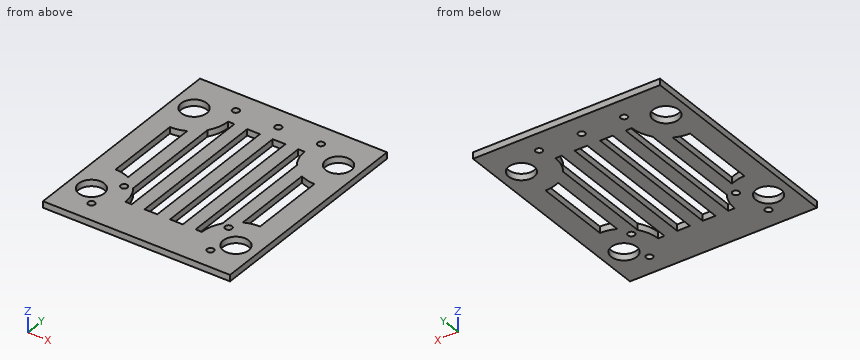
Autodesk Inventor part; units mm, degrees
ref_plane "YZ Plane" through (0, 0, 0) normal (1, 0, 0) x (0, 1, 0)
ref_plane "XZ Plane" through (0, 0, 0) normal (0, 1, 0) x (-1, 0, 0)
ref_plane "XY Plane" through (0, 0, 0) normal (0, 0, 1) x (1, 0, 0)
sketch "スケッチ1" plane through (0, 0, 0) normal (0, 0, 1) x (1, 0, 0)
  line L0 (-22, -24) -> (22, -24)
  line L1 (22, -24) -> (22, 24)
  line L2 (22, 24) -> (-22, 24)
  line L3 (-22, 24) -> (-22, -24)
  line L4 (-22, -24) -> (22, 24) construction
  line L5 (22, -24) -> (-22, 24) construction
  line L6 (-17, 15) -> (17, 15)
  line L7 (17, 15) -> (17, -19)
  line L8 (17, -19) -> (-17, -19)
  line L9 (-17, -19) -> (-17, 15)
  circle A0 centre (-17, 15) radius 3
  circle A1 centre (17, 15) radius 3
  circle A2 centre (17, -19) radius 3
  circle A3 centre (-17, -19) radius 3
  circle A4 centre (-17, 15) radius 8
  circle A5 centre (17, 15) radius 8
  circle A6 centre (17, -19) radius 8
  circle A7 centre (-17, -19) radius 8
  line L10 (-22, -24) -> (22, -24)
  line L11 (22, -24) -> (22, -28)
  line L12 (22, -28) -> (-22, -28)
  line L13 (-22, -28) -> (-22, -24)
  line L14 (-1.5, 15) -> (1.5, 15)
  line L15 (1.5, 15) -> (1.5, -19)
  line L16 (1.5, -19) -> (-1.5, -19)
  line L17 (-1.5, -19) -> (-1.5, 15)
  line L18 (7.5, 15) -> (7.5, -19)
  line L19 (4.5, -19) -> (4.5, 15)
  line L20 (13.5, 15) -> (13.5, -19)
  line L21 (10.5, -19) -> (10.5, 15)
  line L22 (-4.5, 15) -> (-4.5, -19)
  line L23 (-7.5, -19) -> (-7.5, 15)
  line L24 (1.5, 15) -> (1.5, -19)
  line L25 (-1.5, -19) -> (-1.5, 15)
  line L26 (7.5, 15) -> (7.5, -19)
  line L27 (4.5, -19) -> (4.5, 15)
  line L28 (-10.5, 15) -> (-10.5, -19)
  line L29 (-13.5, -19) -> (-13.5, 15)
  line L30 (-4.5, 15) -> (-4.5, -19)
  line L31 (-7.5, -19) -> (-7.5, 15)
  line L32 (1.5, 15) -> (1.5, -19)
  line L33 (-1.5, -19) -> (-1.5, 15)
  point P0 (0, 0)
  point P1 (-9, 15)
  point P2 (9, 15)
  point P3 (17, 7)
  point P4 (17, -11)
  point P5 (9, -19)
  point P6 (-9, -19)
  point P7 (-17, -11)
  point P8 (-17, 7)
  point P9 (22, -24)
  point P10 (0, 15)
  point P11 (-13.5, 7.8063)
  point P12 (-13.5, -11.8063)
  point P13 (-10.5, -14.3363)
  point P14 (-10.5, 10.3363)
  point P15 (10.5, 10.3363)
  point P16 (10.5, -14.3363)
  point P17 (13.5, -11.8063)
  point P18 (13.5, 7.8063)
  dimension "d0" = 48
  dimension "d1" = 44
  dimension "d2" = 34
  dimension "d3" = 5
  dimension "d4" = 5
  dimension "d5" = 6
  dimension "d6" = 16
  dimension "d11" = 4
  dimension "d12" = 3
  dimension "d15" = 6
  dimension "d18" = 6
extrude "プレート1" add sketch "スケッチ1" along normal blind 1.5 contours L3 A7 L9 A3 L8 L0 | L0 A7 L13 | A7 L8 A6 L0 | L0 A6 L11 L12 L13 A7 | L3 A4 L9 A7 | A6 L8 A2 L7 L1 L0 | L0 L11 A6 | L8 L28 A7 | L3 A4 L6 A0 L9 | A7 L29 L8 A3 L9 | A6 L21 L8 | L23 L6 L22 L8 | L8 L29 A7 L28 | A7 L29 A4 L28 | L3 L2 L1 A5 L6 A4 | L9 A0 L6 L29 A4 | A6 L7 A5 L1 | L21 A6 L20 L8 | L8 L19 L6 L18 | L21 A5 L20 A6 | L28 L6 A4 | A4 L29 L6 L28 | A5 L7 A1 L6 L1 | L7 A2 L8 L20 A6 | L21 L6 L20 A5 | A5 L6 L21 | L17 L6 L15 L8 | A5 L20 L6 A1 L7
sketch "スケッチ2" plane through (0, 0, 1.5) normal (0, 0, 1) x (1, 0, 0)
  line L0 (11.5, -21.5) -> (11.5, -14.8)
  line L1 (11.5, -21.5) -> (12, -21.5)
  line L2 (12, -21.5) -> (12, -24)
  line L3 (18, -24) -> (14, -24)
  line L4 (18, -14) -> (18, -24) construction
  line L5 (12.3, -14) -> (18, -14)
  circle A0 centre (12.3, -14.8) radius 0.8
  circle A1 centre (14, -23.2) radius 0.8
  line L6 (0, 0) -> (0, -10)
  circle A2 centre (-12.3, -14.8) radius 0.8
  circle A3 centre (-14, -23.2) radius 0.8
  arc A4 (11.5, -14.8) -> (12.3, -14) centre (12.3, -14.8) ccw
  line L7 (14, -24) -> (12, -24)
  circle A5 centre (14, -23.2) radius 0.8
  dimension "d21" = 1.6
  dimension "d22" = 1.6
  dimension "d25" = 2
extrude "切り取り1" cut sketch "スケッチ2" against normal blind 1.5
sketch "スケッチ3" plane through (0, 0, 1.5) normal (0, 0, 1) x (1, 0, 0)
  circle A0 centre (0, 19) radius 0.8
  circle A1 centre (-10, 19) radius 0.8
  circle A2 centre (10, 19) radius 0.8
  line L0 (-22, 24) -> (22, 24)
  point P0 (0, 0)
  point P1 (0, 24)
  dimension "d26" = 1.6
  dimension "d27" = 1.6
  dimension "d28" = 1.6
  dimension "d29" = 5
  dimension "d30" = 10
  dimension "d31" = 10
extrude "切り取り2" cut sketch "スケッチ3" against normal blind 1.5
equation "\"d4\" = d3"
equation "\"d23\" = Thickness"
equation "\"d32\" = Thickness"
equation "\"d10\" = Thickness"
equation "\"BendRadius\" = Thickness"
equation "\"BendReliefWidth\" = Thickness"
equation "\"BendReliefDepth\" = 0.5 * Thickness"
equation "\"CornerReliefSize\" = 4 * Thickness"
equation "\"MinimumRemnant\" = 2 * Thickness"
equation "\"TransitionRadius\" = BendRadius"
equation "\"JacobiRadiusSize\" = BendRadius"
equation "\"GapSize\" = Thickness"
properties part number "board_setter_base" material "アルミニウム 6061"
Geometry: final body of the model. Coordinates: model frame, mm. Coordinates: 2 decimals unless noted, no trailing zeros. Loops run counter-clockwise (first coordinate to the right, second up) from the corner with the lowest first, then second, coordinate; pieces in that order, holes last. Notation, with made-up numbers: (70.25, 60) - (88.25, 60) arc R25 cw to (88.25, 86) - close; hole circle Ø1 at (63, 3.5). An arc over 180 degrees is marked (long way). Put each result on its own line as item: value. Start each with the question number.
Q1. Line query: line 1 (X direction, y = 10, z = 0.2); line 2 (Y direction, x = -14.5, z = 0.45); line 3 (Y direction, x = 0, z = 0.55). Output: solid intervals per line, ascending.
Q2. Cut plane A-A, the plane x = -3.5. Return loops of the section in (y, z).
Q3. Cut plane D-D, the plane x = 18. Return loops of the section in (y, z), and give its area (3 significant figures).
Q4. Cut plane C-C, the plane y = -7. Return loops of the section in (x, z).
Q5. Pin query (flat end, axial travel): pin 1 Ø5.5 at (x, y) = (17, -19) entering from -Z. Return the tip coordinate at first contact, or that it passes through.
Q6. Cut plane B-B, the plane y = -23.2. Return loops of the section in (x, z).
Filled sheet:
1. line 1: -22 to -10.5, -7.5 to -4.5, -1.5 to 1.5, 4.5 to 7.5, 10.5 to 22
1. line 2: -28 to -23.82, -22.58 to -20.66, -17.34 to -11.4, 7.4 to 13.34, 16.66 to 24
1. line 3: -28 to 18.2, 19.8 to 24
2. outline: (-28, 0) - (-19, 0) - (-19, 1.5) - (-28, 1.5) - close; (15, 0) - (24, 0) - (24, 1.5) - (15, 1.5) - close
3. outline: (-28, 0) - (-21.83, 0) - (-21.83, 1.5) - (-28, 1.5) - close; (-16.17, 0) - (12.17, 0) - (12.17, 1.5) - (-16.17, 1.5) - close; (17.83, 0) - (24, 0) - (24, 1.5) - (17.83, 1.5) - close
3. area: 61.0 mm²
4. outline: (-22, 0) - (-17, 0) - (-17, 1.5) - (-22, 1.5) - close; (-13.5, 0) - (-10.5, 0) - (-10.5, 1.5) - (-13.5, 1.5) - close; (-7.5, 0) - (-4.5, 0) - (-4.5, 1.5) - (-7.5, 1.5) - close; (-1.5, 0) - (1.5, 0) - (1.5, 1.5) - (-1.5, 1.5) - close; (4.5, 0) - (7.5, 0) - (7.5, 1.5) - (4.5, 1.5) - close; (10.5, 0) - (13.5, 0) - (13.5, 1.5) - (10.5, 1.5) - close; (17, 0) - (22, 0) - (22, 1.5) - (17, 1.5) - close
5. pin 1: through
6. outline: (-22, 0) - (-14.8, 0) - (-14.8, 1.5) - (-22, 1.5) - close; (-13.2, 0) - (13.2, 0) - (13.2, 1.5) - (-13.2, 1.5) - close; (14.8, 0) - (22, 0) - (22, 1.5) - (14.8, 1.5) - close
